```python
from build123d import *

# Parameters (mm, degrees)
SKETCH1_W           = 30
SKETCH1_H           = 35
BOSS_EXTRUDE2_DEPTH = 3
SKETCH3_W           = 4
SKETCH3_H           = 35
BOSS_EXTRUDE3_DEPTH = 55
SKETCH4_R           = 1.575
CUT_EXTRUDE2_DEPTH  = 55
FILLET1_R           = 10
SKETCH5_R           = 11
CUT_EXTRUDE3_DEPTH  = 2
SKETCH6_R           = 5
CUT_EXTRUDE4_DEPTH  = 2
FILLET2_R           = 3


with BuildPart() as part:
    # Sketch1 → Boss-Extrude2 (new body)
    with BuildSketch(Plane.XY):
        Rectangle(SKETCH1_W, SKETCH1_H)
    extrude(amount=BOSS_EXTRUDE2_DEPTH)

    # Sketch3 → Boss-Extrude3 (add)
    with BuildSketch(Plane.XY.offset(3)):
        Rectangle(SKETCH3_W, SKETCH3_H)
    extrude(amount=BOSS_EXTRUDE3_DEPTH)

    # Sketch4 → Cut-Extrude2 (cut)
    with BuildSketch(Plane.XY.offset(3)):
        with Locations((10, 10)):
            Circle(SKETCH4_R)
        with Locations((10, -10)):
            Circle(SKETCH4_R)
        with Locations((-10, -10)):
            Circle(SKETCH4_R)
        with Locations((-10, 10)):
            Circle(SKETCH4_R)
    extrude(amount=-CUT_EXTRUDE2_DEPTH, mode=Mode.SUBTRACT)

    # Fillet1
    fillet1_edges = [part.edges().sort_by_distance(p)[0] for p in [
        (0, 17.5, 58),
        (0, -17.5, 58),
        (15, -17.5, 1.5),
        (-15, -17.5, 1.5),
        (-15, 17.5, 1.5),
        (15, 17.5, 1.5),
    ]]
    fillet(fillet1_edges, radius=FILLET1_R)

    # Sketch5 → Cut-Extrude3 (cut)
    with BuildSketch(Plane.ZY.offset(2)):
        with Locations(Location((43, 0, 0), (0, 0, 270))):
            Circle(SKETCH5_R)
    extrude(amount=-CUT_EXTRUDE3_DEPTH, mode=Mode.SUBTRACT)

    # Sketch6 → Cut-Extrude4 (cut)
    with BuildSketch(Plane.ZY):
        with Locations(Location((43, 0, 0), (0, 0, 270))):
            Circle(SKETCH6_R)
    extrude(amount=-CUT_EXTRUDE4_DEPTH, mode=Mode.SUBTRACT)

    # Fillet2
    fillet2_edges = [part.edges().sort_by_distance(p)[0] for p in [
        (2, 0, 3),
        (-2, 0, 3),
    ]]
    fillet(fillet2_edges, radius=FILLET2_R)


solid = part.part
```
Design review of the part built by this model. Coordinates are the model's own, in mm. A direction names the side the tool comes from. Coordinates: 2 decimals unless noted, no trailing zeros. Write each loop counter-clockwise with the first axis right and the second up, starting at its lowest first coordinate (ties: lowest second). Pieces come first, ordered by that corner, then holes. Notation, with made-up numbers: M 9,69 L 15,69 A12 cw 15,86 Z; hole C 33,-25.75 d4. An arc over 180 degrees is marked long. Answer as a JSON object with one key per item and string values.
Item 1: Machinability: for faces 4 (the cylindrical face through (-1.014, 1.432, 53.906)), 5 (the flat face through (15, 0, 1)), 6 (the flat face through (-10, 0, 3)), 7 (the flat face through (2, 0, 32)), which of the approach directions +Z, -Z, +X, -X, +Y, -Y give a long, thin tool a straight path to every point of the face, cutting with its end or side? Answer none if there is none.
Outcome:
{"face 4": "-X", "face 5": "+Z, -Z, +X, +Y, -Y", "face 6": "+Z, -X, +Y, -Y", "face 7": "+Z, +X, +Y, -Y"}
Item 2: Add section C-C, the plane z = 40.5. Give the boundary of the cut face in (x, y).
Outcome:
{"outline": "M -2,-17.5 L 2,-17.5 L 2,-4.33 L 0,-4.33 L 0,-10.71 L -2,-10.71 Z; M -2,10.71 L 0,10.71 L 0,4.33 L 2,4.33 L 2,17.5 L -2,17.5 Z"}
Item 3: Add section A-A, the plane y = 0. Give the boundary of the cut face in (x, z), and give its area (3 significant figures).
Outcome:
{"outline": "M -15,0 L 15,0 L 15,3 L 5,3 A3 cw 2,6 L 2,38 L 0,38 L 0,32 L -2,32 L -2,6 A3 cw -5,3 L -15,3 Z; M -2,54 L 0,54 L 0,48 L 2,48 L 2,58 L -2,58 Z", "area": "250 mm²"}
Item 4: Add section B-B, the plane x = 10.5. Give the boundary of the cut face in (y, z), and give its area (3 significant figures).
Outcome:
{"outline": "M -15.85,0 L -11.49,0 L -11.49,3 L -15.85,3 Z; M -8.51,0 L 8.51,0 L 8.51,3 L -8.51,3 Z; M 11.49,0 L 15.85,0 L 15.85,3 L 11.49,3 Z", "area": "77.2 mm²"}
Item 5: Draft analysis for pull direction Z (two halves, no side actions). For faces 1 (the cylindrical face through (-12.15, 14.49, 1.52)), 2 (the flat face through (0, -2, 38)), 3 (the flat face through (10, 0, 3)), state which applies: pulls with the +Z half, pulls with the -Z half, needs draft (parallel to the pull), parting line crosses it, or undercut.
Outcome:
{"face 1": "needs draft", "face 2": "undercut", "face 3": "pulls with the +Z half"}
Item 6: Insertion check: pin 1 Ø4 at (x, y) = (-10, -10) entering from +Z; pin 2 Ø17.5 at (y, z) = (7, 43) entering from +X; pin 3 Ø11 at (y, z) = (-5.5, 38.5) entering from -X. Each pin has a flat end and moves straight along its axis. Give the tip position at first contact, or say it passes through.
Outcome:
{"pin 1": "z = 3", "pin 2": "x = 2", "pin 3": "x = -2"}
Item 7: Wall thickness on probe 1 along Y at (x, z) = (-10, 2.25) (3 decimals); probe 2 along Z at (x, y) = (-10, 15); probe 3 along X at (y, z) = (-7.5, 24.5): over which ranges is each line inside the solid? List them lowest first.
Outcome:
{"probe 1": "-16.16 to -11.575, -8.425 to 8.425, 11.575 to 16.16", "probe 2": "0 to 3", "probe 3": "-2 to 2"}
Item 8: Add section D-D, the plane y = -13.5. Give the boundary of the cut face in (x, z), and give its area (3 significant figures).
Outcome:
{"outline": "M -13,0 L 13,0 L 13,3 L 5,3 A3 cw 2,6 L 2,56 L -2,56 L -2,6 A3 cw -5,3 L -13,3 Z", "area": "294 mm²"}
